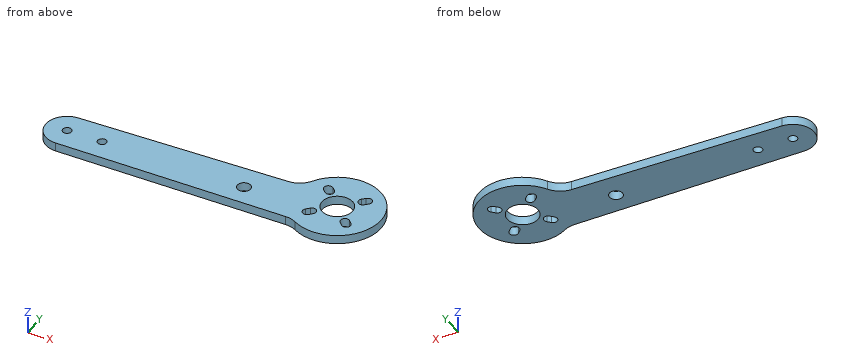
from build123d import *

# Parameters (mm, degrees)
F0_R     = 1
F0_R_2   = 1.5
F0_R_3   = 3.5
F1_DEPTH = 2


# Not quite as in the source:
# - ends of sketch curves that miss each other by under 0.0002 mm in the source are joined


with BuildPart() as f1:
    # F0 (on Top) → F1 (new body)
    with BuildSketch(Plane.XY):
        with BuildLine():
            ThreePointArc((-55.949488929, -12.7158224136), (-54.6584944803, -12.8853634982), (-53.4550506712, -13.3824890802))
            ThreePointArc((-53.4550506712, -13.3824890802), (-38.7798788654, -2.230730151), (-57.0112213811, 0.4786138322))
            ThreePointArc((-57.0112213811, 0.4786138322), (-58.7831707533, -1.2539634751), (-61.1694240668, -1.9228609466))
            Line((-61.1694240668, -1.9228609466), (-108.7206725135, -3.0103658035))
            ThreePointArc((-108.7206725135, -3.0103658035), (-108.7222436347, -3.0104019898), (-108.7238147676, -3.0104376674))
            ThreePointArc((-108.7238147676, -3.0104376674), (-113.4658569564, -7.9179829708), (-108.6128474049, -12.7158224136))
            Line((-108.6128474049, -12.7158224136), (-55.949488929, -12.7158224136))
        make_face()
        with Locations((-108.6128474049, -7.862495663)):
            Circle(F0_R, mode=Mode.SUBTRACT)
        with Locations((-100.6128474049, -7.862495663)):
            Circle(F0_R, mode=Mode.SUBTRACT)
        with Locations((-68.1128474049, -7.862495663)):
            Circle(F0_R_2, mode=Mode.SUBTRACT)
        with BuildLine():
            ThreePointArc((-52.2491954348, -9.9130572553), (-53.6634089972, -9.9130572553), (-53.6634089972, -8.4988436929))
            Line((-53.6634089972, -8.4988436929), (-52.956302216, -7.7917369117))
            ThreePointArc((-52.956302216, -7.7917369117), (-51.5420886536, -7.7917369117), (-51.5420886536, -9.2059504741))
            Line((-51.5420886536, -9.2059504741), (-52.2491954348, -9.9130572553))
        make_face(mode=Mode.SUBTRACT)
        with BuildLine():
            ThreePointArc((-43.2689393138, -8.4988436929), (-43.2689393138, -9.9130572553), (-44.6831528761, -9.9130572553))
            Line((-44.6831528761, -9.9130572553), (-45.3902596573, -9.2059504741))
            ThreePointArc((-45.3902596573, -9.2059504741), (-45.3902596573, -7.7917369117), (-43.9760460949, -7.7917369117))
            Line((-43.9760460949, -7.7917369117), (-43.2689393138, -8.4988436929))
        make_face(mode=Mode.SUBTRACT)
        with Locations((-48.4661741555, -4.7158224136)):
            Circle(F0_R_3, mode=Mode.SUBTRACT)
        with BuildLine():
            ThreePointArc((-53.6634089972, -0.9328011342), (-53.6634089972, 0.4814124282), (-52.2491954348, 0.4814124282))
            Line((-52.2491954348, 0.4814124282), (-51.5420886536, -0.225694353))
            ThreePointArc((-51.5420886536, -0.225694353), (-51.5420886536, -1.6399079154), (-52.956302216, -1.6399079154))
            Line((-52.956302216, -1.6399079154), (-53.6634089972, -0.9328011342))
        make_face(mode=Mode.SUBTRACT)
        with BuildLine():
            ThreePointArc((-43.9760460949, -1.6399079154), (-45.3902596573, -1.6399079154), (-45.3902596573, -0.225694353))
            Line((-45.3902596573, -0.225694353), (-44.6831528761, 0.4814124282))
            ThreePointArc((-44.6831528761, 0.4814124282), (-43.2689393138, 0.4814124282), (-43.2689393138, -0.9328011342))
            Line((-43.2689393138, -0.9328011342), (-43.9760460949, -1.6399079154))
        make_face(mode=Mode.SUBTRACT)
    extrude(amount=F1_DEPTH)


solid = f1.part
CAD build for the part. Positions are in the model's coordinates, mm. Round coordinates to 2 decimals unless told otherwise and drop trailing zeros. Write each loop counter-clockwise with the first axis right and the second up, starting at its lowest first coordinate (ties: lowest second). Pieces come first, ordered by that corner, then holes. Notation, with made-up numbers: M 6,33 L 35,33 A10 cw 35,38 Z; hole C 89.5,9 d11. An arc over 180 degrees is marked long. Use a Markdown table: item, result. Add a question column.
1. Flat gauge pins, fed straight in: P1, Ø4, axis at x = -90, y = -3.5, coming from the -Z side; P2, Ø1.8, axis at x = -108.61, y = -7.86, coming from the +Z side; P3, Ø0.6, axis at x = -80, z = 0.5, coming from the -Y side. Where does each tip first touch, or does it go through?
2. Slice it at C-C on y = -11.5. Give the cut face in (x, z), then the cut area to 3 significant figures.
3. Slice it at D-D on y = 3. Give the cut face in (x, z), then the cut area to 3 significant figures.
4. Slice it at A-A on x = -50. Give the cut face in (y, z), then the cut area to 3 significant figures.
5. Slice it at B-B on z = 1.5. Give the number of separate pieces and of enclosed holes in the cut face, then the cut area to 3 significant figures.
6. Drill centre lines: probe 1 along Y at (x, z) = (-53.5, 1.55); probe 2 along X at (y, z) = (-7, 1.3); probe 3 along X at (y, z) = (-0.25, 0.1). Where is each one in solid material? Low to high.
Reply:
| question | item | result |
|---|---|---|
| 1 | P1 | stops at z = 0 |
| 1 | P2 | passes through |
| 1 | P3 | stops at y = -12.72 |
| 2 | outline | M -111.83,0 L -41.12,0 L -41.12,2 L -111.83,2 Z |
| 2 | area | 141 mm^2 |
| 3 | outline | M -54.83,0 L -42.1,0 L -42.1,2 L -54.83,2 Z |
| 3 | area | 25.4 mm^2 |
| 4 | outline | M -14.6,0 L -7.86,0 L -7.86,2 L -14.6,2 Z; M -1.57,0 L 5.17,0 L 5.17,2 L -1.57,2 Z |
| 4 | area | 26.9 mm^2 |
| 5 | separate pieces | 1 |
| 5 | enclosed holes | 8 |
| 5 | area | 806 mm^2 |
| 6 | probe 1 | y = -13.36 to -10.05, -8.34 to -1.1, 0.61 to 3.92 |
| 6 | probe 2 | x = -113.39 to -109.12, -108.11 to -101.12, -100.11 to -69.34, -66.89 to -51.12, -45.81 to -38.73 |
| 6 | probe 3 | x = -57.55 to -53.96, -51.52 to -45.41, -42.98 to -39.52 |
